Verification items for the finished model (mm, model axes). A direction names the side the tool comes from. Round coordinates to 2 decimals unless told otherwise and drop trailing zeros. Write each loop counter-clockwise with the first axis right and the second up, starting at its lowest first coordinate (ties: lowest second). Pieces come first, ordered by that corner, then holes. Notation, with made-up numbers: M 20,8.5 L 66,8.5 A25 cw 66,46.5 Z; hole C 34.5,31.25 d7. An arc over 180 degrees is marked long. One line per item, written item: value. Start each with the question number.
Item 1: Draft check along Z on faces 3 (the face through (4.437, 0.365, -16.597)), 4 (the face through (4, 19.101, 131)), 5 (the face through (4.437, -0.42, 284.594)), 6 (the face through (4, 16.601, 131)). Enter one of: +Z half, -Z half, draft (parallel to the pull), parting line (faces both ways), or undercut.
Item 2: Section check B-B, the plane y = 0. Record the cut outline in (x, z).
Item 3: Tool access check on faces 1 (the face through (4.437, -0.365, 282.095)), 2 (the face through (9, 17, 133)). Record the directions out of +Z, -Z, +X, -X, +Y, -Y that give a thin tool (end or side, any length) a straight path to the whole face; none if there is none.
Item 4: Gauge pin test, flat ends, axial feed: pin 1 (2 mm diameter, centred on x = 6, y = 13.5, fed in from -Z); pin 2 (4 mm diameter, centred on x = 4.5, y = -5.5, fed in from -Z); pin 3 (1 mm diameter, centred on x = 7.5, y = 1.5, fed in from +Z). Record the tip position at first contact, or that the pin passes through.
Item 5: Section check A-A, the plane x = 7.5. Record the cut outline in (y, z).
Item 6: Section check C-C, the plane z = 98. Record the cut outline in (x, y), then the cut area to 3 significant figures.
Item 7: Thickness scan on probe 1 along Y at (x, z) = (5.25, 161); probe 2 along Z at (x, y) = (2, -3); probe 3 along Z at (x, y) = (3, -4). Record the ranges inside material, lowest first. Write a range as from..to.
Autodesk Inventor part; units mm, degrees
ref_plane "YZ Plane" through (0, 0, 0) normal (1, 0, 0) x (0, 1, 0)
ref_plane "XZ Plane" through (0, 0, 0) normal (0, 1, 0) x (-1, 0, 0)
ref_plane "XY Plane" through (0, 0, 0) normal (0, 0, 1) x (1, 0, 0)
sketch "Sketch1" plane through (0, 0, 0) normal (1, 0, 0) x (0, 1, 0)
  arc A0 (-16.6008, 0) -> (16.6008, 0) centre (0, 0) ccw
  arc A1 (-19.1008, 0) -> (19.1008, 0) centre (0, 0) ccw
  arc A2 (16.6008, 265.4982) -> (-16.6008, 265.4982) centre (0, 265.4982) ccw
  arc A3 (19.1008, 265.4982) -> (-19.1008, 265.4982) centre (0, 265.4982) ccw
  line L0 (16.6008, 0) -> (16.6008, 265.4982)
  line L1 (-16.6008, 0) -> (-16.6008, 265.4982)
  line L2 (19.1008, 0) -> (19.1008, 265.4982)
  line L3 (-19.1008, 0) -> (-19.1008, 265.4982)
  dimension "d0" = 2.5
  dimension "d2" = 265.4982
  dimension "d5" = 19.1008
extrude "Extrusion1" add sketch "Sketch1" along normal blind 9
properties part number "STANDIN,130T,HTD5mm,BELT" material "Nylon 6/6"
Response values:
1. face 3: undercut
1. face 4: draft
1. face 5: +Z half
1. face 6: undercut
2. outline: M 0,-19.1 L 9,-19.1 L 9,-16.6 L 0,-16.6 Z; M 0,282.1 L 9,282.1 L 9,284.6 L 0,284.6 Z
3. face 1: +X, -X
3. face 2: +Z, -Z, +X, +Y, -Y
4. pin 1: stops at z = -14.44
4. pin 2: stops at z = -18.78
4. pin 3: stops at z = 284.57
5. outline: M -19.1,0 A19.1 ccw 19.1,0 L 19.1,265.5 A19.1 ccw -19.1,265.5 Z; hole M -16.6,0 A16.6 ccw 16.6,0 L 16.6,265.5 A16.6 ccw -16.6,265.5 Z
6. outline: M 0,-19.1 L 9,-19.1 L 9,-16.6 L 0,-16.6 Z; M 0,16.6 L 9,16.6 L 9,19.1 L 0,19.1 Z
6. area: 45.0 mm2
7. probe 1: y = -19.1..-16.6, 16.6..19.1
7. probe 2: z = -18.86..-16.33, 281.83..284.36
7. probe 3: z = -18.68..-16.11, 281.61..284.18
